Autodesk Inventor part; units mm, degrees
ref_plane "YZ Plane" through (0, 0, 0) normal (1, 0, 0) x (0, 1, 0)
ref_plane "XZ Plane" through (0, 0, 0) normal (0, 1, 0) x (-1, 0, 0)
ref_plane "XY Plane" through (0, 0, 0) normal (0, 0, 1) x (1, 0, 0)
sketch "Szkic1" plane through (0, 0, 0) normal (0, 0, 1) x (1, 0, 0)
  line L0 (-35.6, 35.6) -> (35.6, 35.6)
  line L1 (35.6, 35.6) -> (35.6, -35.6)
  line L2 (35.6, -35.6) -> (-35.6, -35.6)
  line L3 (-35.6, -35.6) -> (-35.6, 35.6)
  line L4 (-35.6, -35.6) -> (35.6, 35.6) construction
  line L5 (-35.6, 35.6) -> (35.6, -35.6) construction
  line L6 (-30, 30) -> (30, 30) construction
  line L7 (30, 30) -> (30, -30) construction
  line L8 (30, -30) -> (-30, -30) construction
  line L9 (-30, -30) -> (-30, 30) construction
  circle A0 centre (30, 30) radius 3
  circle A1 centre (30, -30) radius 3
  circle A2 centre (-30, -30) radius 3
  circle A3 centre (-30, 30) radius 3
  circle A4 centre (0, 0) radius 28 construction
  line L10 (-11, 13) -> (11, 13)
  line L11 (-10, 10) -> (10, 10)
  line L12 (10, -10) -> (-10, -10)
  line L13 (-4, 4) -> (4, 4)
  line L14 (3.5, 3.2) -> (3.5, -3.2)
  line L15 (4, -4) -> (-3.8927, -4)
  line L16 (-3.5, -3.2) -> (-3.5, 3.2)
  line L17 (4, 4) -> (10, 4)
  line L18 (-4, 4) -> (-10, 4)
  line L19 (-3.8927, -4) -> (-10, -4)
  line L20 (4, -4) -> (10, -4)
  line L21 (-3.5, 3.2) -> (-10, 3.2)
  line L22 (3.5, 3.2) -> (10, 3.2)
  line L23 (-10, -3.2) -> (-3.5, -3.2)
  line L24 (3.5, -3.2) -> (10, -3.2)
  line L25 (10, 10) -> (10, 4)
  line L26 (-10, 4) -> (-10, 10)
  line L27 (-10, -10) -> (-10, -4)
  line L28 (-10, -3.2) -> (-10, 3.2)
  line L29 (10, 3.2) -> (10, -3.2)
  line L30 (10, -4) -> (10, -10)
  line L31 (-12.5, 12.5) -> (-12.5, 25)
  line L32 (12.5, 12.5) -> (12.5, 25)
  line L33 (11, 13) -> (11, 25)
  line L34 (-11, 13) -> (-11, 25)
  line L35 (-11, 25) -> (11, 25)
  line L36 (-12.5, 25) -> (-25, 25)
  line L37 (-25, 25) -> (-25, 0)
  line L38 (12.5, 25) -> (25, 25)
  line L39 (25, 0) -> (25, 25)
  line L40 (-12.5, 12.5) -> (-12.5, 0)
  line L41 (12.5, 12.5) -> (12.5, 0)
  line L42 (-35.6, 0) -> (35.6, 0) construction
  line L43 (-11, -13) -> (11, -13)
  line L44 (-12.5, -12.5) -> (-12.5, -25)
  line L45 (12.5, -12.5) -> (12.5, -25)
  line L46 (11, -13) -> (11, -25)
  line L47 (-11, -13) -> (-11, -25)
  line L48 (-11, -25) -> (11, -25)
  line L49 (-12.5, -25) -> (-25, -25)
  line L50 (-25, -25) -> (-25, 0)
  line L51 (12.5, -25) -> (25, -25)
  line L52 (25, 0) -> (25, -25)
  line L53 (-12.5, -12.5) -> (-12.5, 0)
  line L54 (12.5, -12.5) -> (12.5, 0)
  point P0 (0, 0)
  point P1 (0, 0)
  dimension "d0" = 60
  dimension "d1" = 35.6
  dimension "d2" = 6
  dimension "d3" = 56
  dimension "d4" = 25
  dimension "d5" = 0.8
  dimension "d6" = 0.8
  dimension "d7" = 20
  dimension "d8" = 7
  dimension "d9" = 6
  dimension "d11" = 1.5
  dimension "d12" = 1.5
  dimension "d13" = 25
  dimension "d14" = 12.5
  dimension "d15" = 12.5
  dimension "d16" = 3
extrude "Wyciągnięcie proste1" add sketch "Szkic1" along normal blind 5
sketch "Szkic4" plane through (-35.6, -35.6, 0) normal (0, -1, 0) x (1, 0, 0)
  circle A0 centre (35.6506, 2.5) radius 1.45
  circle A1 centre (35.6506, 2.5) radius 2
  line L0 (0, 0) -> (0, 5) construction
  line L1 (0, 2.5) -> (71.3012, 2.5) construction
  line L2 (39.1, 0) -> (39.1, 5)
  line L3 (34.2012, 4.5) -> (37.1, 4.5)
  line L4 (39.1, 2.5) -> (39.1, 2.5)
  line L5 (37.1, 0.5) -> (34.2012, 0.5)
  line L6 (32.2012, 2.5) -> (32.2012, 2.5)
  line L7 (32.2012, 4.5) -> (39.1, 0.5) construction
  line L8 (39.1, 4.5) -> (32.2012, 0.5) construction
  arc A2 (39.1, 2.5) -> (37.1, 4.5) centre (37.1, 2.5) ccw
  arc A3 (37.1, 0.5) -> (39.1, 2.5) centre (37.1, 2.5) ccw
  arc A4 (32.2012, 2.5) -> (34.2012, 0.5) centre (34.2012, 2.5) ccw
  arc A5 (34.2012, 4.5) -> (32.2012, 2.5) centre (34.2012, 2.5) ccw
  point P0 (35.6, 0)
  dimension "d19" = 2.9
  dimension "d20" = 4
  dimension "d23" = 2
extrude "Wyciągnięcie proste2" cut sketch "Szkic4" against normal blind 26.5 contours A0
extrude "Wyciągnięcie proste3" cut sketch "Szkic4" against normal blind 13 contours A0 | A1 | A1 L3 A2 A3 L5 | A1 L5 A4 A5 L3
sketch "Szkic6" plane through (35.6, -35.6, 0) normal (1, 0, 0) x (0, 0, -1)
  line L0 (0, 71.2) -> (-5, 71.2) construction
  line L1 (-2.5, 71.2) -> (-2.5, 0) construction
  line L2 (0, 0) -> (-5, 0) construction
  circle A0 centre (-2.5, 35.6) radius 1.45
  point P0 (0, 35.6)
  dimension "d26" = 2.9
extrude "Wyciągnięcie proste4" cut sketch "Szkic6" against normal blind 17
sketch "Szkic7" plane through (-35.6, -35.6, 0) normal (-1, 0, 0) x (0, 0, 1)
  line L0 (5, 62.6) -> (0, 62.6)
  circle A0 centre (2.5, 62.6) radius 1
  line L1 (5, 8.6) -> (0, 8.6)
  circle A1 centre (2.5, 8.6) radius 1
  point P0 (0, 35.6)
  dimension "d29" = 2
  dimension "d32" = 2
extrude "Wyciągnięcie proste5" cut sketch "Szkic7" against normal blind 12.25
properties part number "led_holder"
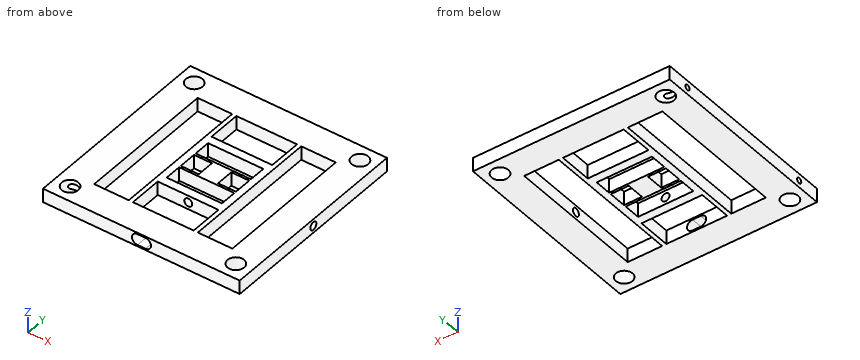
Work out the finished part from the listing and answer in its coordinate system (mm). Give positions to 0.01 mm unless a question says otherwise; leave off trailing zeros. Loops run counter-clockwise (first coordinate to the right, second up) from the corner with the lowest first, then second, coordinate; pieces in that order, holes last. Notation, with made-up numbers: (23, 33.5) -> (47, 33.5) arc R16 ccw to (47, 45.5) -> close; hole circle Ø8 at (17.5, 76.25). An arc over 180 degrees is marked (long way). One line per question, with ' | ' between items. Start each with the question number.
1) Section A-A, the plane y = -30 is taken. Determine the outline of the cut face in (x, z).
2) Each of these flat-tipped pins is pushed along its axis until it touches: pin 1 (1.6 mm diameter, centred on y = -27, z = 2.5, fed in from -X); pin 2 (1.5 mm diameter, centred on x = -5, y = 4.5, fed in from +Z); pin 3 (1.7 mm diameter, centred on y = 0, z = 2.5, fed in from +X); pin 4 (1.5 mm diameter, centred on x = 1, z = 2, fed in from -Y). Where does it stop, or does it pass through?
3) Section C-C, the plane x = 18 is taken. Determine the outline of the cut face in (y, z).
4) Straight lines are drawn through the part: L1, parallel to Y at x = -6, z = 3.4; L2, parallel to X at y = 0.5, z = 4.1; L3, parallel to X at y = 7, z = 2.55. For each, find the intervals that lie inside material, in ascending order.
5) Section D-D, the plane y = -9 is taken. Determine the outline of the cut face in (x, z).
6) Section B-B, the plane x = 30 is taken. Determine the outline of the cut face in (y, z).
Resolved:
1) outline: (-35.6, 0) -> (-33, 0) -> (-33, 5) -> (-35.6, 5) -> close; (-27, 0) -> (27, 0) -> (27, 5) -> (-27, 5) -> close; (33, 0) -> (35.6, 0) -> (35.6, 5) -> (33, 5) -> close; hole (-1.4, 0.5) -> (1.5, 0.5) arc R2 ccw to (1.5, 4.5) -> (-1.4, 4.5) arc R2 ccw to start
2) pin 1: x = -23.35 | pin 2: z = 5 | pin 3: x = 12.5 | pin 4: y = -13
3) outline: (-35.6, 0) -> (-25, 0) -> (-25, 5) -> (-35.6, 5) -> close; (25, 0) -> (35.6, 0) -> (35.6, 5) -> (25, 5) -> close
4) L1: -35.6 to -25, -13 to -10, -4 to -3.2, 3.2 to 4, 10 to 13, 25 to 35.6 | L2: -35.6 to -25, -12.5 to -10, -3.5 to 3.5, 10 to 12.5, 25 to 35.6 | L3: -35.6 to -25, -12.5 to -10, 10 to 12.5, 25 to 35.6
5) outline: (-35.6, 0) -> (-25, 0) -> (-25, 5) -> (-35.6, 5) -> close; (-12.5, 0) -> (-10, 0) -> (-10, 5) -> (-12.5, 5) -> close; (10, 0) -> (12.5, 0) -> (12.5, 5) -> (10, 5) -> close; (25, 0) -> (35.6, 0) -> (35.6, 5) -> (25, 5) -> close
6) outline: (-35.6, 0) -> (-33, 0) -> (-33, 5) -> (-35.6, 5) -> close; (-27, 0) -> (27, 0) -> (27, 5) -> (-27, 5) -> close; (33, 0) -> (35.6, 0) -> (35.6, 5) -> (33, 5) -> close; hole circle Ø2.9 at (0, 2.5)
